Geometry: final body of the model. Coordinates: model frame, mm. Give positions to 0.01 mm unless a question says otherwise; leave off trailing zeros.
from build123d import *

# Parameters (mm, degrees)
F0_R     = 2.1
F1_DEPTH = 406.4


with BuildPart() as f1:
    # F0 (on Front) → F1 (new body)
    with BuildSketch(Plane.XZ):
        with BuildLine():
            Line((-4.64, 10), (-9, 10))
            ThreePointArc((-9, 10), (-9.707107, 9.707107), (-10, 9))
            Line((-10, 9), (-10, 4.64))
            Line((-10, 4.64), (-8.2, 2.84))
            Line((-8.2, 2.84), (-8.2, 5.49934))
            Line((-8.2, 5.49934), (-6.56, 5.49934))
            Line((-6.56, 5.49934), (-3.90066, 2.84))
            Line((-3.90066, 2.84), (-3.90066, 0.15))
            Line((-3.90066, 0.15), (-3.75066, 0))
            Line((-3.75066, 0), (-3.90066, -0.15))
            Line((-3.90066, -0.15), (-3.90066, -2.84))
            Line((-3.90066, -2.84), (-6.56, -5.49934))
            Line((-6.56, -5.49934), (-8.2, -5.49934))
            Line((-8.2, -5.49934), (-8.2, -2.84))
            Line((-8.2, -2.84), (-10, -4.64))
            Line((-10, -4.64), (-10, -9))
            ThreePointArc((-10, -9), (-9.707107, -9.707107), (-9, -10))
            Line((-9, -10), (-4.64, -10))
            Line((-4.64, -10), (-2.84, -8.2))
            Line((-2.84, -8.2), (-5.49934, -8.2))
            Line((-5.49934, -8.2), (-5.49934, -6.56))
            Line((-5.49934, -6.56), (-2.84, -3.90066))
            Line((-2.84, -3.90066), (-0.15, -3.90066))
            Line((-0.15, -3.90066), (0, -3.75066))
            Line((0, -3.75066), (0.15, -3.90066))
            Line((0.15, -3.90066), (2.84, -3.90066))
            Line((2.84, -3.90066), (5.49934, -6.56))
            Line((5.49934, -6.56), (5.49934, -8.2))
            Line((5.49934, -8.2), (2.84, -8.2))
            Line((2.84, -8.2), (4.64, -10))
            Line((4.64, -10), (9, -10))
            ThreePointArc((9, -10), (9.707107, -9.707107), (10, -9))
            Line((10, -9), (10, -4.64))
            Line((10, -4.64), (8.2, -2.84))
            Line((8.2, -2.84), (8.2, -5.49934))
            Line((8.2, -5.49934), (6.56, -5.49934))
            Line((6.56, -5.49934), (3.90066, -2.84))
            Line((3.90066, -2.84), (3.90066, -0.15))
            Line((3.90066, -0.15), (3.75066, 0))
            Line((3.75066, 0), (3.90066, 0.15))
            Line((3.90066, 0.15), (3.90066, 2.84))
            Line((3.90066, 2.84), (6.56, 5.49934))
            Line((6.56, 5.49934), (8.2, 5.49934))
            Line((8.2, 5.49934), (8.2, 2.84))
            Line((8.2, 2.84), (10, 4.64))
            Line((10, 4.64), (10, 9))
            ThreePointArc((10, 9), (9.707107, 9.707107), (9, 10))
            Line((9, 10), (4.64, 10))
            Line((4.64, 10), (2.84, 8.2))
            Line((2.84, 8.2), (5.49934, 8.2))
            Line((5.49934, 8.2), (5.49934, 6.56))
            Line((5.49934, 6.56), (2.84, 3.90066))
            Line((2.84, 3.90066), (0.15, 3.90066))
            Line((0.15, 3.90066), (0, 3.75066))
            Line((0, 3.75066), (-0.15, 3.90066))
            Line((-0.15, 3.90066), (-2.84, 3.90066))
            Line((-2.84, 3.90066), (-5.49934, 6.56))
            Line((-5.49934, 6.56), (-5.49934, 8.2))
            Line((-5.49934, 8.2), (-2.84, 8.2))
            Line((-2.84, 8.2), (-4.64, 10))
        make_face()
        with BuildLine():
            Line((-8.2, -8.2), (-8.2, -6.71))
            ThreePointArc((-8.2, -6.71), (-8.156066, -6.603934), (-8.05, -6.56))
            Line((-8.05, -6.56), (-7.98749, -6.56))
            Line((-7.98749, -6.56), (-6.603934, -7.943556))
            ThreePointArc((-6.603934, -7.943556), (-6.571418, -7.992219), (-6.56, -8.049622))
            Line((-6.56, -8.049622), (-6.56, -8.05))
            ThreePointArc((-6.56, -8.05), (-6.603934, -8.156066), (-6.71, -8.2))
            Line((-6.71, -8.2), (-8.2, -8.2))
        make_face(mode=Mode.SUBTRACT)
        with BuildLine():
            ThreePointArc((6.71, -8.2), (6.603934, -8.156066), (6.56, -8.05))
            Line((6.56, -8.05), (6.56, -7.98749))
            Line((6.56, -7.98749), (7.943556, -6.603934))
            ThreePointArc((7.943556, -6.603934), (7.992219, -6.571418), (8.049622, -6.56))
            Line((8.049622, -6.56), (8.2, -6.56))
            Line((8.2, -6.56), (8.2, -8.05))
            ThreePointArc((8.2, -8.05), (8.156066, -8.156066), (8.05, -8.2))
            Line((8.05, -8.2), (6.71, -8.2))
        make_face(mode=Mode.SUBTRACT)
        with BuildLine():
            ThreePointArc((-8.2, 8.05), (-8.156066, 8.156066), (-8.05, 8.2))
            Line((-8.05, 8.2), (-6.71, 8.2))
            ThreePointArc((-6.71, 8.2), (-6.603934, 8.156066), (-6.56, 8.05))
            Line((-6.56, 8.05), (-6.56, 8.049622))
            ThreePointArc((-6.56, 8.049622), (-6.571418, 7.992219), (-6.603934, 7.943556))
            Line((-6.603934, 7.943556), (-7.943556, 6.603934))
            ThreePointArc((-7.943556, 6.603934), (-7.992219, 6.571418), (-8.049622, 6.56))
            Line((-8.049622, 6.56), (-8.05, 6.56))
            ThreePointArc((-8.05, 6.56), (-8.156066, 6.603934), (-8.2, 6.71))
            Line((-8.2, 6.71), (-8.2, 8.05))
        make_face(mode=Mode.SUBTRACT)
        Circle(F0_R, mode=Mode.SUBTRACT)
        with BuildLine():
            Line((8.2, 8.05), (8.2, 6.71))
            ThreePointArc((8.2, 6.71), (8.156066, 6.603934), (8.05, 6.56))
            Line((8.05, 6.56), (7.98749, 6.56))
            Line((7.98749, 6.56), (6.56, 7.98749))
            Line((6.56, 7.98749), (6.56, 8.05))
            ThreePointArc((6.56, 8.05), (6.603934, 8.156066), (6.71, 8.2))
            Line((6.71, 8.2), (8.05, 8.2))
            ThreePointArc((8.05, 8.2), (8.156066, 8.156066), (8.2, 8.05))
        make_face(mode=Mode.SUBTRACT)
    extrude(amount=F1_DEPTH)


solid = f1.part
Item 1: Section query A-A on y = -28.5. Give the number of separate pieces and of enclosed holes in the cut face, plus the area to 3 significant figures.
Values follow:
separate pieces: 1
enclosed holes: 5
area: 164 mm2
Item 2: Pin query (flat end, axial travel): pin 1 (3 mm diameter, centred on x = 2.5, y = -135.5, fed in from -Z); pin 2 (3 mm diameter, centred on x = -0.5, y = -197.5, fed in from +Z); pin 3 (2 mm diameter, centred on y = -120.5, z = -2.5, fed in from +X). Return the tip coordinate at first contact, or that it passes through.
Values follow:
pin 1: stops at z = -9.36
pin 2: stops at z = 3.9
pin 3: stops at x = 8.86
Item 3: Ray query, probe 1 along X at (y, z) = (-290, 8); probe 2 along Z at (x, y) = (0, -213.5); probe 3 along X at (y, z) = (-188, 3). Return the intervals inside material, ascending.
Values follow:
probe 1: x = -10 to -8.2, -6.57 to -5.5, 5.5 to 6.56, 8.2 to 10
probe 2: z = -3.75 to -2.1, 2.1 to 3.75
probe 3: x = -8.36 to -8.2, -4.06 to 4.06, 8.2 to 8.36
